Part model, mm, in its own coordinate system. A direction names the side the tool comes from. Give positions to 0.01 mm unless a question says otherwise; leave off trailing zeros. Order: outer loops, then holes, each group sorted by start corner. A loop starts at its lowest first (then second) coordinate and runs counter-clockwise, first axis right, second up. Notation, with made-up numbers: M -37,47 L 16,47 A32 cw 16,77 Z; hole C 61.5,-12.75 d3. An arc over 180 degrees is marked long. One line per question, with ' | ' between items.
```python
from build123d import *

# Parameters (mm, degrees)
ESQUISSE1_W           = 29
ESQUISSE1_H           = 29
BOSS_EXTRU_1_DEPTH    = 10
TROU_TARAUD_M32_D     = 2.5
TROU_TARAUD_M32_DEPTH = 8.5
TROU_TARAUD_M32_TIP   = 0.751075774
CONG_2_R              = 2
CONG_1_R              = 1


with BuildPart() as part:
    # Esquisse1 → Boss.-Extru.1 (new body)
    with BuildSketch(Plane.XY):
        Rectangle(ESQUISSE1_W, ESQUISSE1_H)
    extrude(amount=BOSS_EXTRU_1_DEPTH)

    # Trou taraudé M32
    with Locations(Plane(origin=(0, 0, 0), x_dir=(-1, 0, 0), z_dir=(0, 0, -1))):
        with Locations((-11, 11), (11, -11)):
            Hole(TROU_TARAUD_M32_D / 2, depth=TROU_TARAUD_M32_DEPTH)
            with Locations((0, 0, -(TROU_TARAUD_M32_DEPTH + TROU_TARAUD_M32_TIP / 2))):  # 118° drill point
                Cone(0, TROU_TARAUD_M32_D / 2, TROU_TARAUD_M32_TIP, mode=Mode.SUBTRACT)

    # Congé 2
    cong_2_edges = [part.edges().sort_by_distance(p)[0] for p in [
        (-14.5, 14.5, 5),
        (14.5, 14.5, 5),
        (14.5, -14.5, 5),
        (-14.5, -14.5, 5),
    ]]
    fillet(cong_2_edges, radius=CONG_2_R)

    # Congé1
    cong_1_edges = [part.edges().sort_by_distance(p)[0] for p in [
        (0, -14.5, 0),
        (0, -14.5, 10),
        (-14.5, 0, 0),
        (0, 14.5, 0),
        (14.5, 0, 0),
        (-13.914213562, 13.914213562, 0),
        (13.914213562, 13.914213562, 0),
        (13.914213562, -13.914213562, 0),
        (-13.914213562, -13.914213562, 0),
        (-14.5, 0, 10),
        (14.5, 0, 10),
        (0, 14.5, 10),
        (-13.914213562, 13.914213562, 10),
        (13.914213562, 13.914213562, 10),
        (13.914213562, -13.914213562, 10),
        (-13.914213562, -13.914213562, 10),
    ]]
    fillet(cong_1_edges, radius=CONG_1_R)


solid = part.part
```
1. Mould opens along X. For faces 3 (the conical face through (10.8, 10.92, 9.12)), 4 (the cylindrical face through (14.199, 0.175, 9.715)), 5 (the cylindrical face through (-14.199, -0.175, 9.715)) say: released by +X, released by -X, zero draft, split by the parting line, or undercut.
Worked out:
face 3: undercut | face 4: released by +X | face 5: released by -X
2. Probe L1, parallel to X at y = -11, z = 2; L2, parallel to X at y = 11, z = 2.25. List the from-to ranges inside material, lowest first. Write a range as from..to.
Worked out:
L1: x = -14.5..-12.25, -9.75..14.5 | L2: x = -14.5..9.75, 12.25..14.5
3. Slice it at A-A on z = 5.75. Give the cut face in (x, y), then the cut area to 3 significant figures.
Worked out:
outline: M -14.5,-12.5 A2 ccw -12.5,-14.5 L 12.5,-14.5 A2 ccw 14.5,-12.5 L 14.5,12.5 A2 ccw 12.5,14.5 L -12.5,14.5 A2 ccw -14.5,12.5 Z; hole C -11,-11 d2.5; hole C 11,11 d2.5 | area: 828 mm2
4. Tool access for faces 1 (the cylindrical face through (13.9, -13.93, 5.06)), 2 (the cylindrical face through (-11.921, -10.155, 4.31)): list every direction of +Z, -Z, +X, -X, +Y, -Y with a clear straight run to the whole face (end or side of a thin tool).
Worked out:
face 1: +Z, -Z, +X, -Y | face 2: -Z
5. Drop a flat-ended pin along its axis: pin 1 (3 mm diameter, centred on x = -11, y = -11, fed in from -Z). Give the stop position or say it passes through.
Worked out:
pin 1: stops at z = 0
